Can you work these out from the model? Positions are in its coordinate system, mm. Coordinates: 2 decimals unless noted, no trailing zeros. Loops run counter-clockwise (first coordinate to the right, second up) from the corner with the lowest first, then second, coordinate; pieces in that order, holes last.
Autodesk Inventor part; units mm, degrees
ref_plane "XZ Plane" through (0, 0, 0) normal (0, 1, 0) x (-1, 0, 0)
ref_plane "XY Plane" through (0, 0, 0) normal (0, 0, 1) x (1, 0, 0)
sketch "Sketch1" plane through (0, 0, 0) normal (0, 1, 0) x (-1, 0, 0)
  circle A0 centre (0, 0) radius 25
  dimension "d0" = 50
extrude "Extrusion1" add sketch "Sketch1" along normal blind 570
sketch "Sketch2" plane through (0, 0, 0) normal (0, -1, 0) x (1, 0, 0)
  line L0 (-25, -25) -> (25, -25)
  line L1 (25, -25) -> (25, 25)
  line L2 (25, 25) -> (-25, 25)
  line L3 (-25, 25) -> (-25, -25)
  point P0 (0, 0)
extrude "Extrusion2" add sketch "Sketch2" along normal blind 60
sketch "Sketch3" plane through (0, 0, 0) normal (1, 0, 0) x (0, 1, 0)
  circle A0 centre (-30, 0) radius 15
  line L0 (0, -25) -> (0, 0)
  line L1 (0, 25) -> (-60, 25)
  line L2 (0, -25) -> (-60, -25)
  arc A1 (-30, 25) -> (-30, -25) centre (-30, 0) ccw
  line L3 (-30, 25) -> (-30, 40.1158)
  line L4 (-30, 40.1158) -> (-76.6193, 40.1158)
  line L5 (-76.6193, 40.1158) -> (-77.4473, -45.6375)
  line L6 (-77.4473, -45.6375) -> (-35.1048, -45.6375)
  line L7 (-35.1048, -45.6375) -> (-30, -25)
  dimension "d5" = 30
  dimension "d6" = 30
extrude "Extrusion3" cut sketch "Sketch3" along normal mid plane 100
fillet "Fillet1" radius 24.9775 6 edges at (25, -55, 0) (25, -15, -25) (25, -15, 25) (-25, -55, 0) (-25, -15, -25) (-25, -15, 25)
properties part number "Piston_Bom"
Item 1: I'm going to push flat-ended pins straight in: P1, Ø10, axis at y = 63, z = 17.5, coming from the -X side; P2, Ø3, axis at x = -15, y = 199.5, coming from the +Z side; P3, Ø1, axis at x = 0.5, z = -9.5, coming from the -Y side. Where does each tip first touch, or does it pass through?
Results are:
P1: stops at x = -21.65
P2: stops at z = 21.04
P3: stops at y = -53.32
Item 2: We'd pull the mould along Y, two halves only. Please class faces 1 (the face through (0.35, -16.144, -5.745)), 2 (the face through (0, 570, 0)), 3 (the face through (-23.846, 281.01, -7.509)): +Y half, -Y half, draft (parallel to the pull), parting line (faces both ways), or undercut.
Results are:
face 1: undercut
face 2: +Y half
face 3: draft
Item 3: I need wall thicknesses on line 1 along Y through (x, z) = (0.5, 0); line 2 along Y through (x, z) = (-14, 0); line 3 along Z through (x, y) = (3, -30). Which ranges of each line are inside material? Lowest first, please.
Results are:
line 1: y = -55 to -45, -15 to 570
line 2: y = -50.72 to -45, -15 to 570
line 3: z = -24.82 to -15, 15 to 24.82
Item 4: Suppose I cut it at A-A, the plane y = 491. Please give me the cut outline in (x, z), plus the area to 3 significant figures.
Results are:
outline: circle Ø50 at (0, 0)
area: 1,960 mm2
